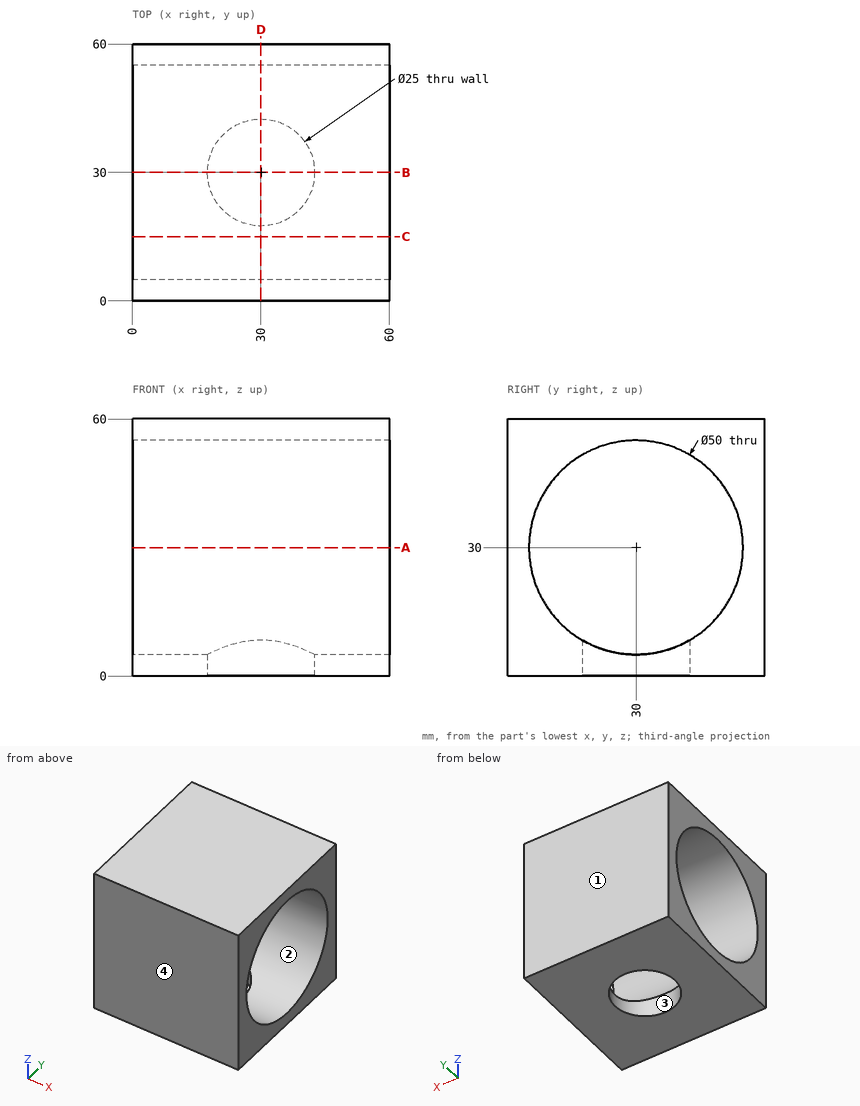
Geometry check sheet. Reference: drawing and pictorial views, mm from the part's lowest x, y, z. Coordinates: 2 decimals unless noted, no trailing zeros. Write each loop counter-clockwise with the first axis right and the second up, starting at its lowest first coordinate (ties: lowest second). Pieces come first, ordered by that corner, then holes. Notation, with made-up numbers: (76.25, 21.25) - (102.25, 21.25) arc R21 ccw to (102.25, 57.25) - close; hole circle Ø4 at (-9.5, 67). An arc over 180 degrees is marked (long way). One line per question, with ' | ' between items. Start each with the question number.
1. Material ranges on line 1 along X through (y, z) = (30, 2.75); line 2 along Z through (x, y) = (36, 30), recorded low to high.
2. Section check A-A (z = 30). Enter the section's corners in (x, y).
3. Draft check along Y on the marked faces 1, 2, 3 and 4. Enter one of: released by +Y, released by -Y, zero draft, split by the parting line, or undercut.
4. Gauge pin test, flat ends, axial feed: P1, Ø22.5, axis at x = 30, y = 30, coming from the -Z side; P2, Ø5, axis at x = 25, z = 22.5, coming from the -Y side. Record the tip position at first contact, or that the pin passes through.
5. Section check B-B (y = 30). Enter the section's corners in (x, z).
6. Section check D-D (x = 30). Enter the section's corners in (y, z), plus the area to 3 significant figures.
7. Section check C-C (y = 15). Enter the section's corners in (x, z).
Computed values:
1) line 1: 0 to 17.5, 42.5 to 60 | line 2: 55 to 60
2) outline: (0, 0) - (60, 0) - (60, 5) - (0, 5) - close; (0, 55) - (60, 55) - (60, 60) - (0, 60) - close
3) face 1: released by +Y | face 2: undercut | face 3: undercut | face 4: released by -Y
4) P1: z = 52.33 | P2: y = 0
5) outline: (0, 0) - (17.5, 0) - (17.5, 5) - (0, 5) - close; (0, 55) - (60, 55) - (60, 60) - (0, 60) - close; (42.5, 0) - (60, 0) - (60, 5) - (42.5, 5) - close
6) outline: (0, 0) - (17.5, 0) - (17.5, 8.35) arc R25 cw (long way) to (42.5, 8.35) - (42.5, 0) - (60, 0) - (60, 60) - (0, 60) - close | area: 1,480 mm²
7) outline: (0, 0) - (60, 0) - (60, 10) - (0, 10) - close; (0, 50) - (60, 50) - (60, 60) - (0, 60) - close
